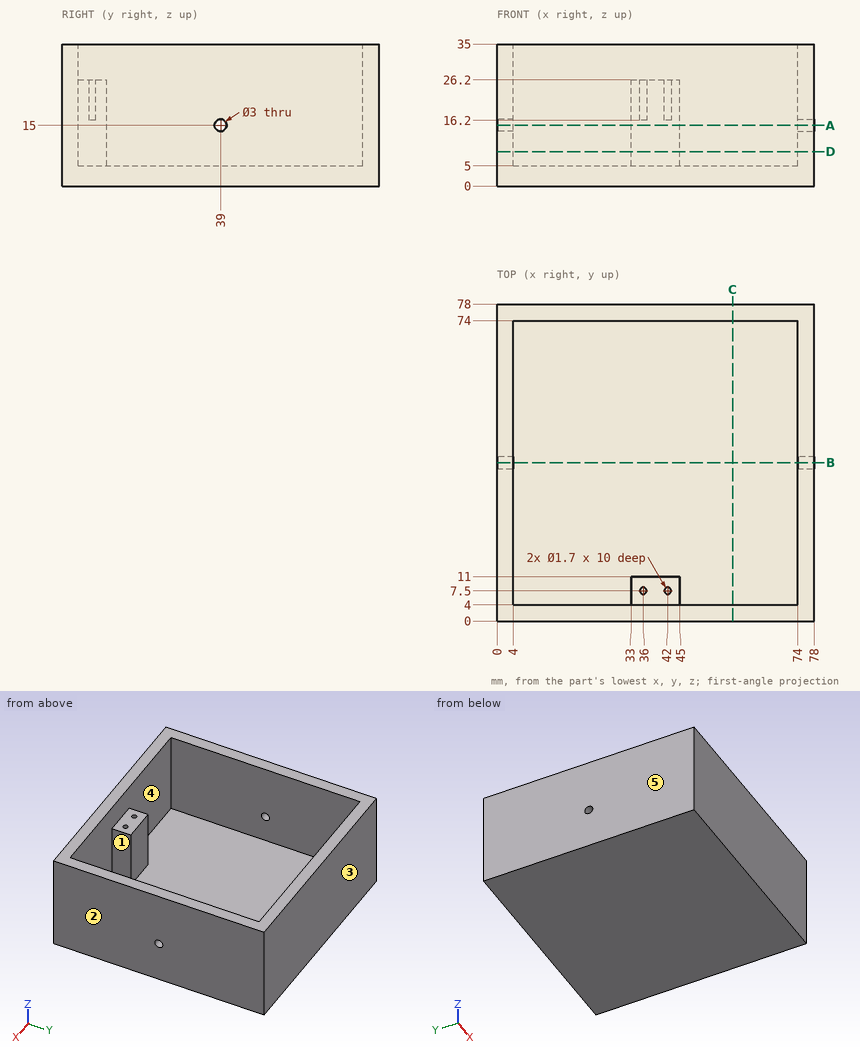
Geometry: see drawing. Coordinates: mm, zero at the bounding-box minimum. A direction names the side the tool comes from. Round coordinates to 2 decimals unless told otherwise and drop trailing zeros. Write each loop counter-clockwise with the first axis right and the second up, starting at its lowest first coordinate (ties: lowest second). Pieces come first, ordered by that corner, then holes.
1) Cut plane B-B (y = 39). Return the cut outline in (x, z), then the cut area to 3 significant figures.
2) Cut plane C-C (x = 58). Return the cut outline in (y, z), then the cut area to 3 significant figures.
3) Cut plane A-A (z = 15). Return the cut outline in (x, y).
4) Ray query, L1, parallel to Y at x = 36, z = 21; L2, parallel to X at y = 68, z = 13.5; L3, parallel to X at y = 7, z = 22. Return the intervals inside material, ascending.
5) Draft query along Y for the marked faces 3, 4 and 5. Return one class per face: pulls with the +Y half, pulls with the -Y half, needs draft (parallel to the pull), parting line crosses it, or undercut.
6) Reachability of the marked faces 1 and 2 from +Z, -Z, +X, -X, +Y, -Y: full face, straight path, thin tool, end or side. Return the list, or none.
7) Contact query for flat-ended pins moving along their axis: P1, Ø2, axis at x = 42, y = 7.5, coming from the +Z side; P2, Ø4, axis at x = 8, y = 15.5, coming from the +Z side; P3, Ø0.5, axis at x = 42.5, y = 7.5, coming from the +Z side. Output: stop coordinate, or through.
8) Cut plane D-D (z = 8.5). Return the cut outline in (x, y).
Geometry says:
1. outline: (0, 0) - (78, 0) - (78, 13.5) - (74, 13.5) - (74, 5) - (4, 5) - (4, 13.5) - (0, 13.5) - close; (0, 16.5) - (4, 16.5) - (4, 35) - (0, 35) - close; (74, 16.5) - (78, 16.5) - (78, 35) - (74, 35) - close
1. area: 606 mm2
2. outline: (0, 0) - (78, 0) - (78, 35) - (74, 35) - (74, 5) - (4, 5) - (4, 35) - (0, 35) - close
2. area: 630 mm2
3. outline: (0, 0) - (78, 0) - (78, 37.5) - (74, 37.5) - (74, 4) - (45, 4) - (45, 11) - (33, 11) - (33, 4) - (4, 4) - (4, 37.5) - (0, 37.5) - close; (0, 40.5) - (4, 40.5) - (4, 74) - (74, 74) - (74, 40.5) - (78, 40.5) - (78, 78) - (0, 78) - close
4. L1: y = 0 to 6.65, 8.35 to 11, 74 to 78
4. L2: x = 0 to 4, 74 to 78
4. L3: x = 0 to 4, 33 to 35.31, 36.69 to 41.31, 42.69 to 45, 74 to 78
5. face 3: pulls with the +Y half
5. face 4: undercut
5. face 5: needs draft
6. face 1: +Z
6. face 2: +Z, -Z, +X, +Y, -Y
7. P1: stops at z = 26.2
7. P2: stops at z = 5
7. P3: stops at z = 16.2
8. outline: (0, 0) - (78, 0) - (78, 78) - (0, 78) - close; hole (4, 4) - (33, 4) - (33, 11) - (45, 11) - (45, 4) - (74, 4) - (74, 74) - (4, 74) - close
